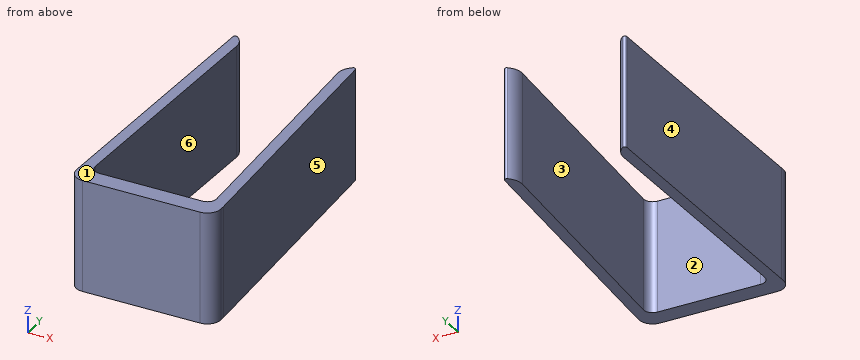
from build123d import *

# Parameters (mm, degrees)
F1_DEPTH    = 25
F2_T1_DEPTH = 44.0569346235
F3_R        = 0.5
F4_R        = 3
F5_R        = 2


# Not quite as in the source:
# - a fillet or chamfer that OpenCascade refuses, or shapes differently, is made with other operations: its cross-section is extruded or revolved along the edge and cut away or added


with BuildPart() as f1:
    # F0 (on Top) → F1 (new body)
    with BuildSketch(Plane.XY):
        Polygon((-13.5, 61.9478940414), (-16, 2), (-13.5, 2), (-11, 61.9478940414), align=None)
        Polygon((13.5, 2), (16, 2), (13.5, 61.9478940414), (11, 61.9478940414), align=None)
        Polygon((-16, -2), (16, -2), (16, 2), (13.5, 2), (-13.5, 2), (-16, 2), align=None)
    extrude(amount=F1_DEPTH)

    # F2: fillet of radius 4 on 2 edges, made by hand

    # F2_s2 → F2_t1 (cut)
    with BuildSketch(Plane.XY.offset(-9.5284673118)):
        with BuildLine():
            ThreePointArc((13.5, 61.9478940414), (11.7478065256, 60.4014195424), (11.1588077885, 58.1398170495))
            Line((11.1588077885, 58.1398170495), (11, 61.9478940414))
            Line((11, 61.9478940414), (13.5, 61.9478940414))
        make_face()
        with BuildLine():
            ThreePointArc((-13.5, 61.9478940414), (-11.7478065256, 60.4014195424), (-11.1588077885, 58.1398170495))
            Line((-11.1588077885, 58.1398170495), (-11, 61.9478940414))
            Line((-11, 61.9478940414), (-13.5, 61.9478940414))
        make_face()
    extrude(amount=F2_T1_DEPTH, mode=Mode.SUBTRACT)

    # F3
    f3_edges = [f1.edges().sort_by_distance(p)[0] for p in [
        (-13.5, 61.947894, 12.5),
        (13.5, 61.947894, 12.5),
    ]]
    fillet(f3_edges, radius=F3_R)

    # F4
    f4_edges = [f1.edges().sort_by_distance(p)[0] for p in [
        (16, -2, 12.5),
        (-16, -2, 12.5),
    ]]
    fillet(f4_edges, radius=F4_R)

    # F5
    f5_edges = [f1.edges().sort_by_distance(p)[0] for p in [
        (-13.5, 2, 12.5),
        (13.5, 2, 12.5),
    ]]
    fillet(f5_edges, radius=F5_R)


solid = f1.part
Verification items for the finished model (mm, model axes). Face numbers are marked on the shaded views. A direction names the side the tool comes from. Round coordinates to 2 decimals unless told otherwise and drop trailing zeros. Loops run counter-clockwise (first coordinate to the right, second up) from the corner with the lowest first, then second, coordinate; pieces in that order, holes last. Notation, with made-up numbers: (31, 13.5) - (61, 13.5) arc R22 ccw to (61, 21.5) - close; hole circle Ø2 at (-8, -2). An arc over 180 degrees is marked (long way). Use a Markdown table: item, result. Add a question column.
1. Section check A-A, the plane y = 9.5. Record the boundary of the cut face in (x, z).
2. Section check B-B, the plane z = 23.75. Record the boundary of the cut face in (x, y).
3. Release check for a two-part mould opening along X. For the marked faces 1, 2, 3 and 4 record: released by +X, released by -X, zero draft, split by the parting line, or undercut.
4. Access from +Z, -Z, +X, -X, +Y, -Y to the whole of each face (thin tool, end or side, straight path). Record for the marked faces 5 and 6.
5. Thickness scan on probe 1 along Y at (x, z) = (-7.5, 7); probe 2 along X at (y, z) = (42, 18.75); probe 3 along X at (y, z) = (47.5, 23.5). Record the ranges inside material, lowest first. Write a range as [from, to].
6. Section check C-C, the plane x = -10. Record the boundary of the cut face in (y, z).
7. Section check D-D, the plane y = 3. Record the boundary of the cut face in (x, z).
8. Gauge pin test, flat ends, axial feed: pin 1 (3 mm diameter, centred on y = 29.5, z = 21, fed in from +X); pin 2 (1.5 mm diameter, centred on y = 45.5, z = 12, fed in from -X); pin 3 (11.5 mm diameter, centred on x = 1, z = 12, fed in from +Y); pin 4 (4 mm diameter, centred on x = 4, y = 5, fed in from -Z). Record the tip position at first contact, or that the pin passes through.
Checks:
| question | item | result |
|---|---|---|
| 1 | outline | (-15.69, 0) - (-13.19, 0) - (-13.19, 25) - (-15.69, 25) - close; (13.19, 0) - (15.69, 0) - (15.69, 25) - (13.19, 25) - close |
| 2 | outline | (-16, 1) arc R3 ccw to (-13, -2) - (13, -2) arc R3 ccw to (16, 1) - (16, 2) - (13.53, 61.11) arc R0.5 ccw to (12.73, 61.49) arc R4 ccw to (11.16, 58.14) - (13.41, 4.08) arc R2 cw to (11.41, 2) - (-11.41, 2) arc R2 cw to (-13.41, 4.08) - (-11.16, 58.14) arc R4 ccw to (-12.73, 61.49) arc R0.5 ccw to (-13.53, 61.11) - (-16, 2) - close |
| 3 | face 1 | zero draft |
| 3 | face 2 | undercut |
| 3 | face 3 | undercut |
| 3 | face 4 | released by -X |
| 4 | face 5 | +Z, -Z, +X, +Y |
| 4 | face 6 | +Z, -Z |
| 5 | probe 1 | y = [-2, 2] |
| 5 | probe 2 | x = [-14.33, -11.83], [11.83, 14.33] |
| 5 | probe 3 | x = [-14.1, -11.6], [11.6, 14.1] |
| 6 | outline | (-2, 0) - (2, 0) - (2, 25) - (-2, 25) - close |
| 7 | outline | (-15.96, 0) - (-13.15, 0) - (-13.15, 25) - (-15.96, 25) - close; (13.15, 0) - (15.96, 0) - (15.96, 25) - (13.15, 25) - close |
| 8 | pin 1 | stops at x = 14.92 |
| 8 | pin 2 | stops at x = -14.22 |
| 8 | pin 3 | stops at y = 2 |
| 8 | pin 4 | passes through |
